Model file for the job. Use its own axes, mm. Face numbers are marked on the shaded views. A direction names the side the tool comes from. Round coordinates to 2 decimals unless told otherwise and drop trailing zeros. Loops run counter-clockwise (first coordinate to the right, second up) from the corner with the lowest first, then second, coordinate; pieces in that order, holes last. Notation, with made-up numbers: M 1,6.25 L 34,6.25 A26 cw 34,20.25 Z; hole C -10.75,46.5 d5. An arc over 180 degrees is marked long. Answer in a Markdown table with one row per item.
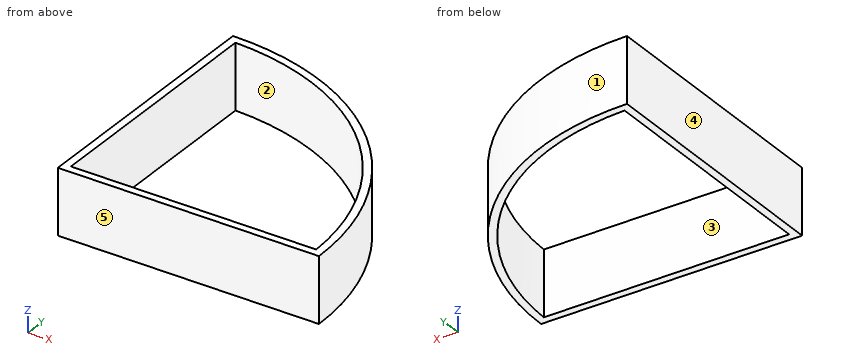
from build123d import *

# Parameters (mm, degrees)
F1_DEPTH = 25
F2_T     = -3
F3_DEPTH = 25


with BuildPart() as f1:
    # F0 (on Top) → F1 (new body)
    with BuildSketch(Plane.XY):
        with BuildLine():
            Line((0, 100), (0, 0))
            Line((0, 0), (100, 0))
            ThreePointArc((100, 0), (70.7106781187, 70.7106781187), (0, 100))
        make_face()
    extrude(amount=-F1_DEPTH)

    # F2
    f2_openings = [f1.faces().sort_by_distance(p)[0] for p in [
        (42.441318, 42.441318, 0),
    ]]
    offset(amount=F2_T, openings=f2_openings)

    # F3 (cut): a face of the model
    f3_faces = [f1.faces().sort_by_distance(p)[0] for p in [
        (42.4961878284, 42.4961878284, -22),
    ]]
    extrude(f3_faces, amount=-F3_DEPTH, mode=Mode.SUBTRACT)


solid = f1.part
1. Saw through at A-A (x = 62). Write the cut outline in (y, z).
Verdict:
| item | result |
|---|---|
| outline | M 0,-25 L 3,-25 L 3,0 L 0,0 Z; M 74.6,-25 L 78.46,-25 L 78.46,0 L 74.6,0 Z |
2. Pin check, flat tips, straight feed: pin 1 (8 mm diameter, centred on y = 42.5, z = -5, fed in from +X); pin 2 (1.5 mm diameter, centred on y = 57, z = -5, fed in from +X); pin 3 (6 mm diameter, centred on y = 82, z = -7.5, fed in from +X). Stop position of each tip, or through.
Verdict:
| item | result |
|---|---|
| pin 1 | stops at x = 92.29 |
| pin 2 | stops at x = 82.68 |
| pin 3 | stops at x = 61.31 |
3. Saw through at C-C (z = -22.25). Write the cut outline in (x, y).
Verdict:
| item | result |
|---|---|
| outline | M 0,0 L 100,0 A100 ccw 0,100 Z; hole M 3,3 L 96.95,3 A97 ccw 3,96.95 Z |
4. Mould opens along Y. For the marked faces 3, 4 and 5 say: +Y half, -Y half, draft (parallel to the pull), parting line (faces both ways), or undercut.
Verdict:
| item | result |
|---|---|
| face 3 | undercut |
| face 4 | draft |
| face 5 | -Y half |
5. Wall check: probe 1 along Y at (x, z) = (46, -9); probe 2 along X at (y, z) = (66.5, -19); probe 3 along X at (y, z) = (5.5, -4). Give the ranges that are in metal, low to high.
Verdict:
| item | result |
|---|---|
| probe 1 | y = 0 to 3, 85.4 to 88.79 |
| probe 2 | x = 0 to 3, 70.62 to 74.68 |
| probe 3 | x = 0 to 3, 96.84 to 99.85 |
6. Saw through at B-B (y = 39). Write the cut outline in (x, z).
Verdict:
| item | result |
|---|---|
| outline | M 0,-25 L 3,-25 L 3,0 L 0,0 Z; M 88.81,-25 L 92.08,-25 L 92.08,0 L 88.81,0 Z |
7. Tool access for the marked faces 1 and 2: list every direction of +Z, -Z, +X, -X, +Y, -Y with a clear straight run to the whole face (end or side of a thin tool).
Verdict:
| item | result |
|---|---|
| face 1 | +Z, -Z, +X, +Y |
| face 2 | +Z, -Z |
